Read the model definition and answer for the solid it produces. Units are mm, in the model's axes. Give positions to 0.01 mm unless a question says otherwise; leave off trailing zeros. Order: outer loops, then holes, each group sorted by start corner. A loop starts at its lowest first (then second) coordinate and runs counter-clockwise, first axis right, second up. Notation, with made-up numbers: (-20, -14.75) -> (29, -14.75) arc R24 ccw to (29, 23.25) -> close; hole circle Ø1 at (80, 44.25). An arc over 180 degrees is marked (long way). One line per question, with ' | ' between items. Start each with the question number.
Solid Edge part; units mm, degrees
sketch "Sketch1" plane through (-12.9316, 0, 8.7363) normal (0, -1, 0) x (1, 0, 0)
  line L0 (16.6581, 7.5929) -> (14.5325, 7.5929)
  line L1 (7.4081, -11.0071) -> (14.5325, 7.5929)
  line L2 (7.4081, -11.0071) -> (8.4081, -11.0071)
  line L3 (16.6581, 7.5929) -> (8.4081, -11.0071)
extrude "Protrusion1" add sketch "Sketch1" along normal blind 4
sketch "Sketch2" plane through (-12.9316, 0, 8.7363) normal (0, -1, 0) x (1, 0, 0)
  line L0 (14.5325, 7.5929) -> (14.8919, 8.5313)
  line L1 (34.4273, 9.2134) -> (14.8919, 8.5313)
  line L2 (34.4273, 8.2134) -> (34.4273, 9.2134)
  line L3 (16.6581, 7.5929) -> (34.4273, 8.2134)
extrude "Protrusion2" add sketch "Sketch2" along normal blind 4 material side at (1.8273, 0, 16.7805)
sketch "Sketch3" plane through (-12.9316, 0, 8.7363) normal (0, -1, 0) x (1, 0, 0)
  line L0 (14.5325, 7.5929) -> (14.8919, 8.5313)
  line L1 (34.4273, 9.2134) -> (14.8919, 8.5313)
  line L2 (34.4273, 8.2134) -> (34.4273, 9.2134)
  line L3 (16.6581, 7.5929) -> (34.4273, 8.2134)
extrude "Protrusion3" add sketch "Sketch3" against normal blind 13.75 material side at (1.8273, 0, 16.7805)
sketch "Sketch4" plane through (11.7448, 4.4474, 17.6092) normal (-0.0348995, 0, 0.9993908) x (0.9993908, 0, 0.0348995)
  line L0 (9.7568, -8.4474) -> (9.7568, 0.5526)
  line L1 (4.2568, -8.4474) -> (9.7568, 0.5526)
  line L2 (9.7568, -8.4474) -> (4.2568, -8.4474)
extrude "Cutout1" cut sketch "Sketch4" along normal mid plane 3.8186
sketch "Sketch5" plane through (-0.2942, 14.8774, 17.1888) normal (-0.0348995, 0, 0.9993908) x (0.9993908, 0, 0.0348995)
  line L0 (1.8325, -1.1274) -> (12.3325, -1.1274)
  line L1 (12.3325, -1.1274) -> (12.3325, -6.3774)
  line L2 (12.3325, -6.3774) -> (1.8325, -6.3774)
  line L3 (1.8325, -6.3774) -> (1.8325, -1.1274)
extrude "ExtrudedCutout_2" cut sketch "Sketch5" against normal blind 10.4175
properties material "Stainless Steel, 420"
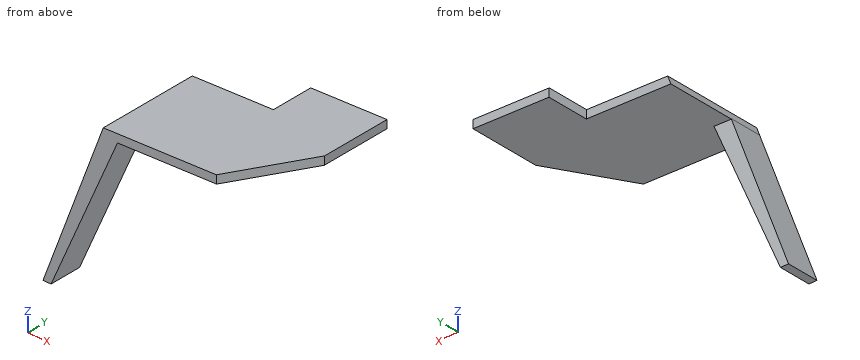
Q1. A cutting plane is placed at B-B, the plane x = 2.75. Determine the outline of the cut face in (y, z).
Q2. A cutting plane is placed at D-D, the plane y = 5.75. Determine the outline of the cut face in (x, z), then the cut area to 3 significant figures.
Q3. Find the intervals of material crossed by line 1 (Y direction, x = -1, z = 8.75); line 2 (Z direction, x = 15, y = 6.5); line 3 (Z direction, x = 19.5, y = 12.75), in increasing order.
Q4. Given P1, Ø8, axis at y = 3.5, z = 11.5, coming from the -X side; P2, Ø3, axis at x = 0, z = 7.5, coming from the +Y side; P3, Ø8, axis at x = 10.5, y = 3.5, coming from the +Z side, each flat-ended and moving along its own axis, determine where each tip first touches the part or whether it passes through.
Q5. A cutting plane is placed at C-C, the plane z = 2.5. Determine the outline of the cut face in (x, y), then the cut area to 3 significant figures.
Q6. A cutting plane is placed at A-A, the plane y = -2. Determine the outline of the cut face in (x, z), then the cut area to 3 significant figures.
Geometry results:
1) outline: (-4, 14.13) -> (0, 14.13) -> (0, 16.3) -> (8.5, 16.3) -> (8.5, 17.3) -> (-4, 17.3) -> close
2) outline: (1.57, 16.25) -> (21.5, 16.95) -> (21.5, 17.95) -> (1.96, 17.27) -> close | area: 19.7 mm²
3) line 1: -4 to 0 | line 2: 16.72 to 17.72 | line 3: 16.88 to 17.88
4) P1: x = -0.99 | P2: y = 0 | P3: z = 17.71
5) outline: (-3.7, -4) -> (-2.41, -4) -> (-2.41, 0) -> (-3.7, 0) -> close | area: 5.15 mm²
6) outline: (-5.52, -2.27) -> (-4.52, -2.27) -> (3.73, 16.33) -> (17.26, 16.8) -> (17.22, 17.8) -> (1.96, 17.27) -> (1.6, 16.33) -> close | area: 44.5 mm²
